from build123d import *

# Parameters (mm, degrees)
SKETCH1_W           = 56
SKETCH1_H           = 40
BOSS_EXTRUDE1_DEPTH = 4
SKETCH3_W           = 56
SKETCH3_H           = 3
CUT_EXTRUDE2_DEPTH  = 2
SKETCH4_R           = 1.5
CUT_EXTRUDE3_DEPTH  = 5
SKETCH5_W           = 56
SKETCH5_H           = 3
BOSS_EXTRUDE2_DEPTH = 2


with BuildPart() as part:
    # Sketch1 → Boss-Extrude1 (new body)
    with BuildSketch(Plane.XY):
        with Locations((28, 20)):
            Rectangle(SKETCH1_W, SKETCH1_H)
    extrude(amount=BOSS_EXTRUDE1_DEPTH)

    # Sketch3 → Cut-Extrude2 (cut)
    with BuildSketch(Plane.XY.offset(4)):
        with Locations((28, 1.5)):
            Rectangle(SKETCH3_W, SKETCH3_H)
    extrude(amount=-CUT_EXTRUDE2_DEPTH, mode=Mode.SUBTRACT)

    # Sketch4 → Cut-Extrude3 (cut, through all)
    with BuildSketch(Plane.XY.offset(4)):
        with Locations((47.5, 5)):
            Circle(SKETCH4_R)
        with Locations((30, 5)):
            Circle(SKETCH4_R)
        with Locations((12.5, 5)):
            Circle(SKETCH4_R)
        with Locations((47.5, 35)):
            Circle(SKETCH4_R)
        with Locations((30, 35)):
            Circle(SKETCH4_R)
        with Locations((12.5, 35)):
            Circle(SKETCH4_R)
    extrude(amount=-CUT_EXTRUDE3_DEPTH, mode=Mode.SUBTRACT)

    # Sketch5 → Boss-Extrude2 (add)
    with BuildSketch(Plane.XY.offset(4)):
        with Locations((28, 1.5)):
            Rectangle(SKETCH5_W, SKETCH5_H)
    extrude(amount=-BOSS_EXTRUDE2_DEPTH)


solid = part.part
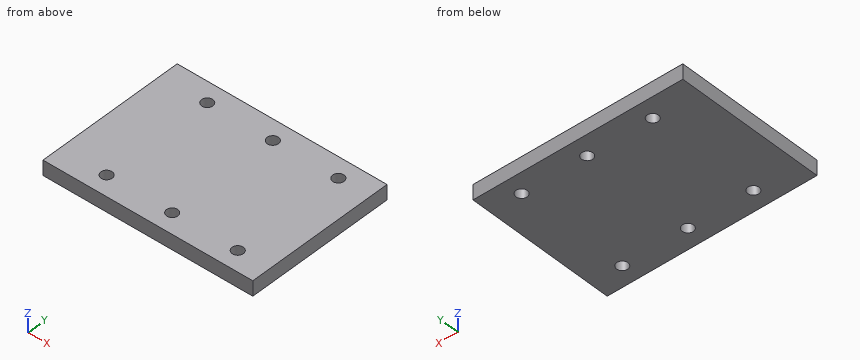
CAD build for the part. Positions are in the model's coordinates, mm. Round coordinates to 2 decimals unless told otherwise and drop trailing zeros. Order: outer loops, then holes, each group sorted by start corner. A loop starts at its lowest first (then second) coordinate and runs counter-clockwise, first axis right, second up. Notation, with made-up numbers: (56.5, -5) -> (90.5, -5) arc R31 cw to (90.5, 33) -> close; hole circle Ø1 at (-6.75, -19.75). An arc over 180 degrees is marked (long way). Write each question's results on one line, items separated by ' | '.
1. Cut at B-B (x = 12.5). Give the cut face in (y, z).
Findings below:
outline: (0, 0) -> (3.5, 0) -> (3.5, 4) -> (0, 4) -> close; (6.5, 0) -> (33.5, 0) -> (33.5, 4) -> (6.5, 4) -> close; (36.5, 0) -> (40, 0) -> (40, 4) -> (36.5, 4) -> close
2. Cut at C-C (z = 1.75). Give the cut face in (x, y), plus the area to 3 significant figures.
Findings below:
outline: (0, 0) -> (56, 0) -> (56, 40) -> (0, 40) -> close; hole circle Ø3 at (12.5, 5); hole circle Ø3 at (12.5, 35); hole circle Ø3 at (30, 5); hole circle Ø3 at (30, 35); hole circle Ø3 at (47.5, 5); hole circle Ø3 at (47.5, 35) | area: 2,200 mm²
3. Cut at A-A (y = 5). Give the cut face in (x, z), plus the area to 3 significant figures.
Findings below:
outline: (0, 0) -> (11, 0) -> (11, 4) -> (0, 4) -> close; (14, 0) -> (28.5, 0) -> (28.5, 4) -> (14, 4) -> close; (31.5, 0) -> (46, 0) -> (46, 4) -> (31.5, 4) -> close; (49, 0) -> (56, 0) -> (56, 4) -> (49, 4) -> close | area: 188 mm²
4. Flat gauge pin, fed straight in: P1, Ø5, axis at x = 30, y = 35, coming from the -Z side. Where does the tip first touch, or does it go through?
Findings below:
P1: stops at z = 0
5. Wall check: line 1 along Y through (x, z) = (47.5, 1.95); line 2 along X through (y, z) = (34.5, 3). Give the ranges that are in metal, low to high. Write a range as [from, to].
Findings below:
line 1: y = [0, 3.5], [6.5, 33.5], [36.5, 40] | line 2: x = [0, 11.09], [13.91, 28.59], [31.41, 46.09], [48.91, 56]
